Geometry check sheet. Reference: the model listing, model coordinates, mm. Face numbers are marked on the shaded views. A direction names the side the tool comes from. Round coordinates to 2 decimals unless told otherwise and drop trailing zeros. Order: outer loops, then holes, each group sorted by start corner. A loop starts at its lowest first (then second) coordinate and runs counter-clockwise, first axis right, second up.
(1) Sectioned sample at B-B (y = 23.5). Record the boundary of the cut face in (x, z).
(2) Sectioned sample at D-D (y = 37.5). Record the boundary of the cut face in (x, z).
(3) Set-up check for the marked faces 4 and 5: record each of +Z, -Z, +X, -X, +Y, -Y from which the full face is reachable in a straight line by a thin tool's end or side.
(4) Material ranges on line 1 along Y through (x, z) = (-75, 55); line 2 along X through (y, z) = (2, 25); line 3 along X through (y, z) = (40, 27.5), recorded low to high.
(5) Sectioned sample at C-C (z = -25). Record the boundary of the cut face in (x, y).
(6) Release check for a two-part mould opening along Z. For the marked faces 1, 2 and 3 record: +Z half, -Z half, draft (parallel to the pull), parting line (faces both ways), or undercut.
(7) Sectioned sample at A-A (x = -94). Record the boundary of the cut face in (y, z), plus the area to 3 significant figures.
(8) Go/stop test with flat-tipped pins: pin 1 (1.2 mm diameter, centred on x = 76, y = 37, fed in from +Z); pin 2 (9 mm diameter, centred on y = 33, z = 10, fed in from -X); pin 3 (2 mm diameter, centred on x = -75.5, z = -25.5, fed in from -Y). Record where each tip stops, or that it passes through.
from build123d import *

# Parameters (mm, degrees)
SKETCH1_W           = 215
SKETCH1_H           = 115
BOSS_EXTRUDE1_DEPTH = 50
SKETCH2_W           = 20
SKETCH2_H           = 111
CUT_EXTRUDE1_DEPTH  = 30
SKETCH3_R           = 2
CUT_EXTRUDE2_DEPTH  = 5
SKETCH4_R           = 2
CUT_EXTRUDE3_DEPTH  = 3


with BuildPart() as part:
    # Sketch1 → Boss-Extrude1 (new body)
    with BuildSketch(Plane(origin=(0, 0, 0), x_dir=(1, 0, 0), z_dir=(0, 1, 0))):
        Rectangle(SKETCH1_W, SKETCH1_H)
    extrude(amount=BOSS_EXTRUDE1_DEPTH)

    # Sketch2 → Cut-Extrude1 (cut)
    with BuildSketch(Plane(origin=(0, 50, 0), x_dir=(1, 0, 0), z_dir=(0, 1, 0))):
        with Locations((-97.5, 0)):
            Rectangle(SKETCH2_W, SKETCH2_H)
    extrude(amount=-CUT_EXTRUDE1_DEPTH, mode=Mode.SUBTRACT)

    # Sketch3 → Cut-Extrude2 (cut)
    with BuildSketch(Plane.XZ):
        with Locations(Location((-75, 25, 0), (0, 0, 270))):
            Circle(SKETCH3_R)
        with Locations(Location((75, 25, 0), (0, 0, 270))):
            Circle(SKETCH3_R)
        with Locations(Location((75, -25, 0), (0, 0, 270))):
            Circle(SKETCH3_R)
        with Locations(Location((-75, -25, 0), (0, 0, 270))):
            Circle(SKETCH3_R)
    extrude(amount=-CUT_EXTRUDE2_DEPTH, mode=Mode.SUBTRACT)

    # Sketch4 → Cut-Extrude3 (cut)
    with BuildSketch(Plane.XY.offset(57.5)):
        with Locations((-75, 12.5)):
            Circle(SKETCH4_R)
        with Locations((-75, 37.5)):
            Circle(SKETCH4_R)
        with Locations((75, 37.5)):
            Circle(SKETCH4_R)
        with Locations((75, 12.5)):
            Circle(SKETCH4_R)
    extrude(amount=-CUT_EXTRUDE3_DEPTH, mode=Mode.SUBTRACT)


solid = part.part
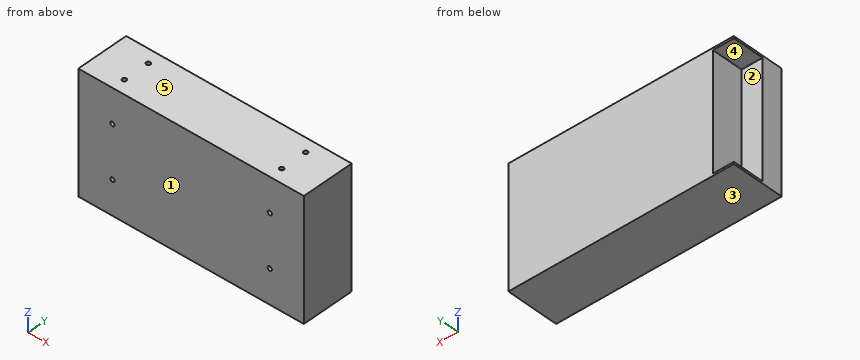
Answer below:
1. outline: (-107.5, -57.5) - (107.5, -57.5) - (107.5, 57.5) - (-107.5, 57.5) - (-107.5, 55.5) - (-87.5, 55.5) - (-87.5, -55.5) - (-107.5, -55.5) - close
2. outline: (-107.5, -57.5) - (107.5, -57.5) - (107.5, 57.5) - (77, 57.5) - (77, 54.5) - (73, 54.5) - (73, 57.5) - (-73, 57.5) - (-73, 54.5) - (-77, 54.5) - (-77, 57.5) - (-107.5, 57.5) - (-107.5, 55.5) - (-87.5, 55.5) - (-87.5, -55.5) - (-107.5, -55.5) - close
3. face 4: -X, +Y
3. face 5: +Z, +X, -X, +Y, -Y
4. line 1: y = 0 to 10.5, 14.5 to 35.5, 39.5 to 50
4. line 2: x = -107.5 to -77, -73 to 73, 77 to 107.5
4. line 3: x = -87.5 to 107.5
5. outline: (-107.5, 0) - (-77, 0) - (-77, 5) - (-73, 5) - (-73, 0) - (73, 0) - (73, 5) - (77, 5) - (77, 0) - (107.5, 0) - (107.5, 50) - (-87.5, 50) - (-87.5, 20) - (-107.5, 20) - close
6. face 1: draft
6. face 2: undercut
6. face 3: -Z half
7. outline: (0, -57.5) - (50, -57.5) - (50, -55.5) - (20, -55.5) - (20, 55.5) - (50, 55.5) - (50, 57.5) - (0, 57.5) - close
7. area: 2,420 mm2
8. pin 1: stops at z = 54.5
8. pin 2: stops at x = -87.5
8. pin 3: stops at y = 5
